from build123d import *

# Parameters (mm, degrees)
F0_R     = 4.25
F1_DEPTH = 3
F2_R     = 4.25
F2_R_2   = 3.5
F3_DEPTH = 2.75
F4_R     = 0.5
F5_DEPTH = 1
F6_SIZE  = 0.1


with BuildPart() as f1:
    # F0 (on Top) → F1 (new body)
    with BuildSketch(Plane.XY):
        Circle(F0_R)
    extrude(amount=F1_DEPTH)

    # F2 (on face) → F3 (join)
    with BuildSketch(Plane.XY.offset(3)):
        Circle(F2_R)
        Circle(F2_R_2, mode=Mode.SUBTRACT)
    extrude(amount=F3_DEPTH)

    # F4 (on face) → F5 (join)
    with BuildSketch(Plane(origin=(0, 0, 0), x_dir=(1, 0, 0), z_dir=(0, 0, -1))):
        with Locations((-2, 0)):
            Circle(F4_R)
        with Locations((2, 0)):
            Circle(F4_R)
    extrude(amount=F5_DEPTH)

    # F6
    f6_edges = [f1.edges().sort_by_distance(p)[0] for p in [
        (-3.5, 0, 5.75),
        (-4.25, 0, 5.75),
    ]]
    chamfer(f6_edges, length=F6_SIZE)


solid = f1.part
Build history of the part. All positions in model axes, mm. A direction names the side the tool comes from. Coordinates: 2 decimals unless noted, no trailing zeros. Write each loop counter-clockwise with the first axis right and the second up, starting at its lowest first coordinate (ties: lowest second). Pieces come first, ordered by that corner, then holes. Notation, with made-up numbers: (37, 79.5) -> (63, 79.5) arc R29 cw to (63, 105.5) -> close; hole circle Ø8 at (-6, 65). An arc over 180 degrees is marked (long way). Use CSV: the item, a comma, the result in double quotes. Start each with the question number.
Q1. Cut at D-D, the plane z = 1. List the corners of the cut face in (x, y).
Q2. Cut at A-A, the plane y = 0. List the corners of the cut face in (x, z), then the cut area to 3 significant figures.
Q3. 3-axis set-ups, long thin cutter, end or side, ignore diameter. For faces 1 (the cylindrical face through (3.233, -1.341, 4.306)), 2 (the cylindrical face through (1.5, 0, -0.5)), 3 (the flat face through (2, 0, -1)): which of +Z, -Z, +X, -X, +Y, -Y reach the whole face in a straight line?
Q4. Pull direction X, two halves, no side cores. Call faces 4 (the cylindrical face through (2.285, 3.584, 2.785)), 5 (the cylindrical face through (-2.4, 0.3, -0.5)), 6 (the flat face through (0, 4, 5.75)): released by +X, released by -X, zero draft, split by the parting line, or undercut.
Q5. Flat gauge pins, fed straight in: pin 1 Ø1 at (y, z) = (3.5, 2) entering from -X; pin 2 Ø4 at (x, z) = (3, 3) entering from +Y; pin 3 Ø1 at (x, y) = (0, 3.5) entering from -Z. Where does each tip first touch, or does it go through?
Q6. Drill centre lines: probe 1 along Y at (x, z) = (0, 4.1); probe 2 along Z at (x, y) = (3.75, -1.5); probe 3 along Z at (x, y) = (-0.5, 2). Where is each one in solid material? Low to high.
Q7. Cut at C-C, the plane z = 3.75. List the corners of the cut face in (x, y), then the cut area to 3 significant figures.
Q8. Cut at B-B, the plane x = 0. List the corners of the cut face in (y, z).
Checked values:
1,outline,"circle Ø8.5 at (0, 0)"
2,outline,"(-4.25, 0) -> (-2.5, 0) -> (-2.5, -1) -> (-1.5, -1) -> (-1.5, 0) -> (1.5, 0) -> (1.5, -1) -> (2.5, -1) -> (2.5, 0) -> (4.25, 0) -> (4.25, 5.65) -> (4.15, 5.75) -> (3.6, 5.75) -> (3.5, 5.65) -> (3.5, 3) -> (-3.5, 3) -> (-3.5, 5.65) -> (-3.6, 5.75) -> (-4.15, 5.75) -> (-4.25, 5.65) -> close"
2,area,"31.6 mm²"
3,face 1,"+Z"
3,face 2,"-Z"
3,face 3,"-Z, +X, -X, +Y, -Y"
4,face 4,"split by the parting line"
4,face 5,"undercut"
4,face 6,"zero draft"
5,pin 1,"stops at x = -3.01"
5,pin 2,"stops at y = 4.13"
5,pin 3,"stops at z = 0"
6,probe 1,"y = -4.25 to -3.5, 3.5 to 4.25"
6,probe 2,"z = 0 to 5.75"
6,probe 3,"z = 0 to 3"
7,outline,"circle Ø8.5 at (0, 0); hole circle Ø7 at (0, 0)"
7,area,"18.3 mm²"
8,outline,"(-4.25, 0) -> (4.25, 0) -> (4.25, 5.65) -> (4.15, 5.75) -> (3.6, 5.75) -> (3.5, 5.65) -> (3.5, 3) -> (-3.5, 3) -> (-3.5, 5.65) -> (-3.6, 5.75) -> (-4.15, 5.75) -> (-4.25, 5.65) -> close"
